The model under review builds one solid part; all positions refer to its coordinate system, in mm. Face numbers are marked on the shaded views. A direction names the side the tool comes from. Coordinates: 2 decimals unless noted, no trailing zeros. Loops run counter-clockwise (first coordinate to the right, second up) from the corner with the lowest first, then second, coordinate; pieces in that order, holes last. Notation, with made-up numbers: (58.25, 53) - (71.25, 53) arc R17 ccw to (71.25, 61) - close; hole circle Ø5 at (-2.75, 87.25). An arc over 180 degrees is marked (long way). Use a Markdown table: item, result. Add a question column.
1) Add section A-A, the plane x = 0. Give the boundary of the cut face in (y, z), and give its area (3 significant figures).
2) Add section D-D, the plane z = 4.75. Give the number of separate pieces and of enclosed holes in the cut face, and give its area (3 significant figures).
3) To check wall thickness, follow L1, parallel to X at y = -11, z = 5.8; L2, parallel to Y at x = 36, z = 3.65; L3, parallel to Y at x = -7.5, z = 2.15. State the ranges of each line that lie inside material, in increasing order. Write a range as [from, to].
4) Add section C-C, the plane y = -10.5. Give the boundary of the cut face in (x, z), and give its area (3 significant figures).
5) Clearance check with a flat-ended pin moving along its axis: pin 1 (3 mm diameter, centred on x = 5.5, z = 1, fed in from -Y). State where the tip first meets the part, or that it passes through.
6) For the marked faces 4, 5 and 6, list the 3-axis set-ups (+Z, -Z, +X, -X, +Y, -Y) from which the entire face can be reached by the end or side of a thin tool; tool diameter is ignored.
7) Add section B-B, the plane y = 0. Give the boundary of the cut face in (x, z).
8) The part is to be moulded in two halves that separate along Y. For the marked faces 1, 2 and 3, say which applies: pulls with the +Y half, pulls with the -Y half, needs draft (parallel to the pull), parting line crosses it, or undercut.
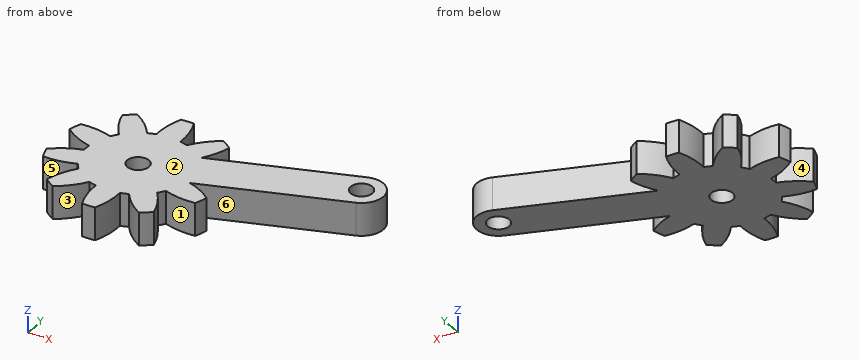
Autodesk Inventor part; units mm, degrees
ref_plane "Work Plane2" through (0, 0, 3) normal (0, 0, 1) x (-1, 0, 0)
ref_plane "Work Plane8" through (0, 0, 0) normal (0.9510565, 0.309017, 0) x (0, 0, 1)
ref_plane "Work Plane9" through (0, 0, 0) normal (1, 0, 0) x (0, 1, 0)
sketch "Sketch1" plane through (0, 0, 0) normal (0, 0, 1) x (1, 0, 0)
  circle A0 centre (0, 0) radius 15.0851
  dimension "d0" = 30.1702
extrude "Extrusion1" add sketch "Sketch1" along normal blind 6
ref_plane "Work Plane2" through (0, 0, 3) normal (0, 0, 1) x (-1, 0, 0)
sketch "Sketch2" plane through (0, 0, 0) normal (0, 0, -1) x (-1, 0, 0)
  circle A0 centre (0, 0) radius 15.0851
  circle A1 centre (0, 0) radius 12.5
  dimension "d3" = 25
surface extrude "Pitch Diameter" sketch "Sketch2" against normal through all shown no curves A1
ref_plane "Work Plane8" through (0, 0, 0) normal (0.9510565, 0.309017, 0) x (0, 0, 1)
ref_plane "Work Plane9" through (0, 0, 0) normal (1, 0, 0) x (0, 1, 0)
spur gear teeth "Spur Gear" teeth 10 pitch diameter 25 tip diameter 30.1702 root diameter 18.9292 face width 6 start plane through (0, 0, 0) normal (0, 0, -1) x (-1, 0, 0)
sketch "Sketch3" plane through (0, 0, 0) normal (0, 0, -1) x (-1, 0, 0)
  circle A0 centre (0, 0) radius 2
  dimension "d49" = 4
extrude "Extrusion2" cut sketch "Sketch3" against normal up to surface (6 mm away)
sketch "Sketch4" plane through (0, 0, 0) normal (0, 0, -1) x (-1, 0, 0)
  circle A0 centre (-26.4586, 35.0672) radius 2
  line L0 (-4.8178, 32.2415) -> (-25.2225, 38.8714)
  arc A1 (-25.2225, 38.8714) -> (-27.6947, 31.263) centre (-26.4586, 35.0672) ccw
  line L1 (-27.6947, 31.263) -> (-7.2899, 24.6331)
  arc A2 (-7.2899, 24.6331) -> (-7.2592, 22.759) centre (7.7794, 23.9426) ccw
  arc A3 (-7.2592, 22.759) -> (-1.4237, 21.7331) centre (-2.0301, 35.3932) ccw
  arc A4 (-1.4237, 21.7331) -> (-0.9647, 20.3206) centre (7.7794, 23.9426) ccw
  arc A5 (-0.9647, 20.3206) -> (-5.0828, 16.0606) centre (6.5738, 8.913) ccw
  arc A6 (-5.0828, 16.0606) -> (-3.6914, 14.1456) centre (7.7794, 23.9426) ccw
  arc A7 (-3.6914, 14.1456) -> (1.6326, 16.7456) centre (-6.8872, 27.4404) ccw
  arc A8 (1.6326, 16.7456) -> (2.8342, 15.8727) centre (7.7794, 23.9426) ccw
  arc A9 (2.8342, 15.8727) -> (2.0066, 10.0058) centre (15.6383, 11.0747) ccw
  arc A10 (2.0066, 10.0058) -> (4.2579, 9.2743) centre (7.7794, 23.9426) ccw
  arc A11 (4.2579, 9.2743) -> (7.0368, 14.5072) centre (-6.1421, 18.1516) ccw
  arc A12 (7.0368, 14.5072) -> (8.522, 14.5072) centre (7.7794, 23.9426) ccw
  arc A13 (8.522, 14.5072) -> (11.301, 9.2743) centre (21.7009, 18.1516) ccw
  arc A14 (11.301, 9.2743) -> (13.5522, 10.0058) centre (7.7794, 23.9426) ccw
  arc A15 (13.5522, 10.0058) -> (12.7247, 15.8727) centre (-0.0794, 11.0747) ccw
  arc A16 (12.7247, 15.8727) -> (13.9262, 16.7456) centre (7.7794, 23.9426) ccw
  arc A17 (13.9262, 16.7456) -> (19.2502, 14.1456) centre (22.446, 27.4404) ccw
  arc A18 (19.2502, 14.1456) -> (20.6416, 16.0606) centre (7.7794, 23.9426) ccw
  arc A19 (20.6416, 16.0606) -> (16.5236, 20.3206) centre (8.985, 8.913) ccw
  arc A20 (16.5236, 20.3206) -> (16.9825, 21.7331) centre (7.7794, 23.9426) ccw
  arc A21 (16.9825, 21.7331) -> (22.818, 22.759) centre (17.589, 35.3932) ccw
  arc A22 (22.818, 22.759) -> (22.818, 25.1262) centre (7.7794, 23.9426) ccw
  arc A23 (22.818, 25.1262) -> (16.9825, 26.1521) centre (17.589, 12.492) ccw
  arc A24 (16.9825, 26.1521) -> (16.5236, 27.5646) centre (7.7794, 23.9426) ccw
  arc A25 (16.5236, 27.5646) -> (20.6416, 31.8246) centre (8.985, 38.9722) ccw
  arc A26 (20.6416, 31.8246) -> (19.2502, 33.7396) centre (7.7794, 23.9426) ccw
  arc A27 (19.2502, 33.7396) -> (13.9262, 31.1396) centre (22.446, 20.4448) ccw
  arc A28 (13.9262, 31.1396) -> (12.7247, 32.0125) centre (7.7794, 23.9426) ccw
  arc A29 (12.7247, 32.0125) -> (13.5522, 37.8794) centre (-0.0794, 36.8105) ccw
  arc A30 (13.5522, 37.8794) -> (11.301, 38.6109) centre (7.7794, 23.9426) ccw
  arc A31 (11.301, 38.6109) -> (8.522, 33.378) centre (21.7009, 29.7336) ccw
  arc A32 (8.522, 33.378) -> (7.0368, 33.378) centre (7.7794, 23.9426) ccw
  arc A33 (7.0368, 33.378) -> (4.2579, 38.6109) centre (-6.1421, 29.7336) ccw
  arc A34 (4.2579, 38.6109) -> (2.0066, 37.8794) centre (7.7794, 23.9426) ccw
  arc A35 (2.0066, 37.8794) -> (2.8342, 32.0125) centre (15.6383, 36.8105) ccw
  arc A36 (2.8342, 32.0125) -> (1.6326, 31.1396) centre (7.7794, 23.9426) ccw
  arc A37 (1.6326, 31.1396) -> (-3.6914, 33.7396) centre (-6.8872, 20.4448) ccw
  arc A38 (-3.6914, 33.7396) -> (-4.8178, 32.2415) centre (7.7794, 23.9426) ccw
  circle A39 centre (7.7794, 23.9426) radius 1.5
  line L2 (-1.2361, -3.8042) -> (-35.4741, 7.3204)
  line L3 (-38.0423, 12.3607) -> (-38.0423, 12.3607)
  line L4 (-33.002, 14.9288) -> (1.2361, 3.8042)
  line L5 (1.2361, 3.8042) -> (-1.2361, -3.8042)
  circle A40 centre (-34.238, 11.1246) radius 2
  arc A41 (-38.0423, 12.3607) -> (-35.4741, 7.3204) centre (-34.238, 11.1246) ccw
  arc A42 (-33.002, 14.9288) -> (-38.0423, 12.3607) centre (-34.238, 11.1246) ccw
  line L6 (-6.619, 6.3565) -> (-9.0911, -1.252)
  point P0 (0, 0)
  point P1 (-36.8062, 16.1649)
  point P2 (-39.2783, 8.5565)
  point P3 (-38.0423, 12.3607)
  dimension "d61" = 40
  dimension "d62" = 8
  dimension "d63" = 4
  dimension "d64" = 0
  dimension "d65" = 4
  dimension "d66" = 4
  dimension "d67" = 4
extrude "Extrusion3" add sketch "Sketch4" against normal up to surface (6 mm away) contours L2 A41 A42 L4 L6
equation "\"d0\" = da_da"
equation "\"d1\" = da_b"
equation "\"d3\" = da_d"
equation "\"d16\" = da_aw"
equation "\"d43\" = da_aw"
equation "\"d46\" = da_aw"
properties part number "Spur Gear2" material "Steel"
From the geometry:
| question | item | result |
|---|---|---|
| 1 | outline | (-15.09, 0) - (-2, 0) - (-2, 6) - (-15.09, 6) - close; (2, 0) - (15.09, 0) - (15.09, 6) - (2, 6) - close |
| 1 | area | 157 mm^2 |
| 2 | separate pieces | 1 |
| 2 | enclosed holes | 2 |
| 2 | area | 691 mm^2 |
| 3 | L1 | x = [-9.67, -5.49], [-2.17, 2.17], [5.49, 9.67] |
| 3 | L2 | y = [7.53, 10.18], [12.07, 14.72] |
| 3 | L3 | y = [-12.62, -6.54], [-5.77, 5.77], [6.54, 12.62] |
| 4 | outline | (-9.53, 0) - (-5, 0) - (-5, 6) - (-9.53, 6) - close; (-2.21, 0) - (2.21, 0) - (2.21, 6) - (-2.21, 6) - close; (5, 0) - (9.53, 0) - (9.53, 6) - (5, 6) - close |
| 4 | area | 80.8 mm^2 |
| 5 | pin 1 | stops at y = -12.27 |
| 6 | face 4 | +Z, -Z, -X |
| 6 | face 5 | +Z, -Z |
| 6 | face 6 | +Z, -Z, +X |
| 7 | outline | (-9.46, 0) - (-2, 0) - (-2, 6) - (-9.46, 6) - close; (2, 0) - (12.94, 0) - (12.94, 6) - (2, 6) - close |
| 8 | face 1 | undercut |
| 8 | face 2 | needs draft |
| 8 | face 3 | pulls with the -Y half |
